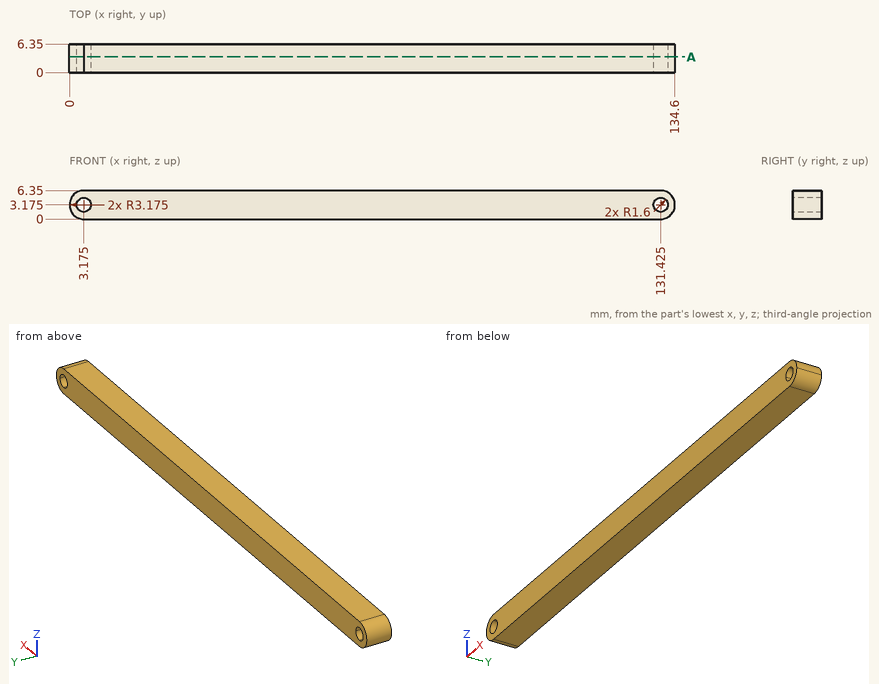
Can you work these out from the drawing? Everything is in mm from the part's minimum corner. Give positions to 0.01 mm unless a question says otherwise; leave off trailing zeros. Put each result on its own line as item: value. Start each with the question number.
(1) Will these pins go through, and if not, where does the flat tip stop? pin 1 Ø1 at (y, z) = (2, 1) entering from +X; pin 2 Ø2 at (y, z) = (0.5, 5.5) entering from -X.
(2) I want a section at A-A on y = 3.5. State how many separate pieces and enclosed holes the cut face has, then the cut area to 3 significant figures.
(3) I need wall thicknesses on line 1 along X through (y, z) = (5.5, 3) (1 decimal); line 2 along X through (y, z) = (4, 1.75) (1 decimal); line 3 along X through (y, z) = (5.5, 5.5). Which ranges of each line are inside material? Lowest first, please. Write a range as [from, to].
Answer block:
1. pin 1: x = 134.12
1. pin 2: x = 0.29
2. separate pieces: 1
2. enclosed holes: 2
2. area: 830 mm^2
3. line 1: [0, 1.6], [4.8, 129.8], [133, 134.6]
3. line 2: [0.3, 2.4], [3.9, 130.7], [132.2, 134.3]
3. line 3: [1.01, 133.59]
